Design review of the part built by this model. Coordinates are the model's own, in mm. A direction names the side the tool comes from. Give positions to 0.01 mm unless a question says otherwise; leave off trailing zeros. Order: outer loops, then holes, each group sorted by start corner. A loop starts at its lowest first (then second) coordinate and runs counter-clockwise, first axis right, second up. Notation, with made-up numbers: (29.5, 12) -> (63.5, 12) arc R22 cw to (63.5, 46) -> close; hole circle Ø2 at (20, 15). An arc over 180 degrees is marked (long way). Return JSON: item names as keys, results as strings.
```python
from build123d import *

# Parameters (mm, degrees)
SKETCH2_W           = 2
SKETCH2_H           = 8.1
BOSS_EXTRUDE1_DEPTH = 20
SKETCH3_W           = 4
SKETCH3_H           = 2
BOSS_EXTRUDE2_DEPTH = 6


with BuildPart() as part:
    # Sketch2 → Boss-Extrude1 (new body)
    with BuildSketch(Plane.XY):
        Polygon((-2.04, 7.95), (0, 7.95), (0, -7.95), (-2.04, -7.95), (-6.152414984, -4.048), (-6.152414984, 4.048), align=None)
        with Locations((1, 0)):
            Rectangle(SKETCH2_W, SKETCH2_H)
    extrude(amount=BOSS_EXTRUDE1_DEPTH)

    # Sketch3 → Boss-Extrude2 (add)
    with BuildSketch(Plane.XY.offset(20)):
        with Locations((-4.152414984, 0)):
            Rectangle(SKETCH3_W, SKETCH3_H)
    extrude(amount=BOSS_EXTRUDE2_DEPTH)


solid = part.part
```
Item 1: Add section B-B (x = -2.5). Give the boundary of the cut face in (y, z).
Result set:
{"outline": "(-7.51, 0) -> (7.51, 0) -> (7.51, 20) -> (1, 20) -> (1, 26) -> (-1, 26) -> (-1, 20) -> (-7.51, 20) -> close"}
Item 2: Add section C-C (y = -0.25). Give the boundary of the cut face in (x, z).
Result set:
{"outline": "(-6.15, 0) -> (2, 0) -> (2, 20) -> (-2.15, 20) -> (-2.15, 26) -> (-6.15, 26) -> close"}
Item 3: Add section D-D (x = -3.75). Give the boundary of the cut face in (y, z).
Result set:
{"outline": "(-6.33, 0) -> (6.33, 0) -> (6.33, 20) -> (1, 20) -> (1, 26) -> (-1, 26) -> (-1, 20) -> (-6.33, 20) -> close"}
Item 4: Add section A-A (z = 2). Give the boundary of the cut face in (x, y).
Result set:
{"outline": "(-6.15, -4.05) -> (-2.04, -7.95) -> (0, -7.95) -> (0, -4.05) -> (2, -4.05) -> (2, 4.05) -> (0, 4.05) -> (0, 7.95) -> (-2.04, 7.95) -> (-6.15, 4.05) -> close"}
Item 5: Machinability: for faces 1 (the face through (1, 4.05, 10)), 2 (the face through (-2.152, 0, 23)), 3 (the face through (1, -4.05, 10)), 4 (the face through (-4, -1, 23)), which of the approach directions +Z, -Z, +X, -X, +Y, -Y give a long, thin tool a straight path to every point of the face, cutting with its end or side? Answer none if there is none.
Result set:
{"face 1": "+Z, -Z, +X, +Y", "face 2": "+Z, +X, +Y, -Y", "face 3": "+Z, -Z, +X, -Y", "face 4": "+Z, +X, -X, -Y"}
Item 6: Wall thickness on L1, parallel to Z at x = 0.5, y = -2; L2, parallel to Y at x = 1.75, z = 8.75; L3, parallel to X at y = -6.75, z = 5.5: over which ranges is each line inside the solid? List them lowest first. Write a range as [from, to].
Result set:
{"L1": "z = [0, 20]", "L2": "y = [-4.05, 4.05]", "L3": "x = [-3.3, 0]"}
Item 7: For pin 1 (1 mm diameter, centred on y = 0, z = 22.5, fed in from +X); pin 2 (2 mm diameter, centred on x = -3.5, z = 24, fed in from -Y); pin 3 (1.6 mm diameter, centred on x = 1, z = 5.5, fed in from +Y), all flat-tipped, find the tip position at first contact; note any pin that passes through.
Result set:
{"pin 1": "stops at x = -2.15", "pin 2": "stops at y = -1", "pin 3": "stops at y = 4.05"}
